The listing builds one solid part. Answer for the finished solid, in the listing's coordinates (mm). Coordinates: 2 decimals unless noted, no trailing zeros. Loops run counter-clockwise (first coordinate to the right, second up) from the corner with the lowest first, then second, coordinate; pieces in that order, holes last. Notation, with made-up numbers: M -14,-29 L 35,-29 A13 cw 35,-13 Z; hole C -11.5,3 d9. An arc over 180 degrees is marked long. Answer as a JSON object with one key per item and string values. Group by question number.
1. A cutting plane is placed at B-B on x = 0. Give the vertices of the cut face in (y, z) (1 decimal).
2. Determine the mould class of faces 1 (the face through (0, 2, 3.175)), 2 (the face through (-0.62, -71.48, 1.61)) for opening direction Y: released by +Y, released by -Y, zero draft, split by the parting line, or undercut.
3. A cutting plane is placed at A-A on y = -76.2. Give the vertices of the cut face in (x, z) (1 decimal).
4. Straight lines are drawn through the part: L1, parallel to Y at x = 0, z = 1.85; L2, parallel to X at y = 76, z = 2; L3, parallel to Y at x = 2, z = 1.25. For each, find the intervals that lie inside material, in ascending order.
Autodesk Inventor part; units mm, degrees
ref_plane "YZ Plane" through (0, 0, 0) normal (1, 0, 0) x (0, 1, 0)
ref_plane "XZ Plane" through (0, 0, 0) normal (0, 1, 0) x (-1, 0, 0)
ref_plane "XY Plane" through (0, 0, 0) normal (0, 0, 1) x (1, 0, 0)
sketch "Sketch1" plane through (0, 0, 0) normal (0, 0, 1) x (1, 0, 0)
  line L0 (-25.4, -127) -> (25.4, -127)
  line L1 (25.4, -127) -> (25.4, 127)
  line L2 (25.4, 127) -> (-25.4, 127)
  line L3 (-25.4, 127) -> (-25.4, -127)
  line L4 (-25.4, -127) -> (25.4, 127) construction
  line L5 (25.4, -127) -> (-25.4, 127) construction
  point P0 (0, 0)
  dimension "d0" = 50.8
  dimension "d1" = 254
extrude "Extrusion1" add sketch "Sketch1" along normal blind 3.175
sketch "Sketch2" plane through (0, 0, 3.175) normal (0, 0, 1) x (1, 0, 0)
  line L0 (25.4, 127) -> (-25.4, 127) construction
  line L1 (0, 127) -> (0, -127) construction
  line L2 (-25.4, -127) -> (25.4, -127) construction
  circle A0 centre (0, 76.2) radius 4.7625
  circle A1 centre (0, -76.2) radius 4.7625
  point P0 (0, 0)
  dimension "d4" = 50.8
  dimension "d5" = 50.8
  dimension "d6" = 9.525
  dimension "d7" = 9.525
extrude "Extrusion2" cut sketch "Sketch2" against normal through all
equation "\"d0\" = basicLiftWidth"
equation "\"d1\" = basicLiftLength"
equation "\"d2\" = basicLiftThickness"
equation "\"d4\" = basicLLiftAxelsDistanceFromTop"
equation "\"d5\" = basicLiftaxelDistancefromBottom"
equation "\"d6\" = baslicLiftAxelDiam"
equation "\"d7\" = baslicLiftAxelDiam"
equation "\"basicLiftLength\" = 254"
equation "\"basicLiftWidth\" = 50.8"
equation "\"basicLiftaxelDistancefromBottom\" = 50.8"
equation "\"basicLLiftAxelsDistanceFromTop\" = 50.8"
equation "\"basicLiftThickness\" = 3.175"
equation "\"baslicLiftAxelDiam\" = 9.525"
properties part number "basicLiftPlate" material "Aluminum 6061"
From the geometry:
{
 "1": {"outline": "M -127,0 L -81,0 L -81,3.2 L -127,3.2 Z; M -71.4,0 L 71.4,0 L 71.4,3.2 L -71.4,3.2 Z; M 81,0 L 127,0 L 127,3.2 L 81,3.2 Z"},
 "2": {"face 1": "zero draft", "face 2": "undercut"},
 "3": {"outline": "M -25.4,0 L -4.8,0 L -4.8,3.2 L -25.4,3.2 Z; M 4.8,0 L 25.4,0 L 25.4,3.2 L 4.8,3.2 Z"},
 "4": {"L1": "y = -127 to -80.96, -71.44 to 71.44, 80.96 to 127", "L2": "x = -25.4 to -4.76, 4.76 to 25.4", "L3": "y = -127 to -80.52, -71.88 to 71.88, 80.52 to 127"}
}
